```python
from build123d import *

# Parameters (mm, degrees)
SKETCH006_W     = 85.5
SKETCH006_H     = 85.5
SKETCH006_W_2   = 73.5
SKETCH006_H_2   = 73.5
PAD003_DEPTH    = 6
SKETCH007_W     = 85.5
SKETCH007_H     = 85.5
SKETCH007_R     = 25.5
PAD004_DEPTH    = 2
SKETCH008_R     = 1.5
POCKET_DEPTH    = 8.001
SKETCH009_R     = 1.5
POCKET001_DEPTH = 5
FILLET002_R     = 3


with BuildPart() as part:
    # Sketch006 → Pad003 (new body)
    with BuildSketch(Plane.XY):
        Rectangle(SKETCH006_W, SKETCH006_H)
        Rectangle(SKETCH006_W_2, SKETCH006_H_2, mode=Mode.SUBTRACT)
    extrude(amount=PAD003_DEPTH)

    # Sketch007 (on Face10 of Pad003) → Pad004 (join)
    with BuildSketch(Plane.XY.offset(6)):
        Rectangle(SKETCH007_W, SKETCH007_H)
        Circle(SKETCH007_R, mode=Mode.SUBTRACT)
    extrude(amount=PAD004_DEPTH)

    # Sketch008 (on Face4 of Pad004) → Pocket (cut, through all)
    with BuildSketch(Plane(origin=(0, 0, 0), x_dir=(1, 0, 0), z_dir=(0, 0, -1))):
        with Locations((-39.235281, 39.235281)):
            Circle(SKETCH008_R)
        with Locations((39.235281, 39.235281)):
            Circle(SKETCH008_R)
        with Locations((39.235281, -39.235281)):
            Circle(SKETCH008_R)
        with Locations((-39.235281, -39.235281)):
            Circle(SKETCH008_R)
    extrude(amount=-POCKET_DEPTH, mode=Mode.SUBTRACT)

    # Sketch009 (on Face17 of Pocket) → Pocket001 (cut)
    with BuildSketch(Plane.XY.offset(8)):
        with Locations((-30, 30)):
            Circle(SKETCH009_R)
        with Locations((30, 30)):
            Circle(SKETCH009_R)
        with Locations((30, -30)):
            Circle(SKETCH009_R)
        with Locations((-30, -30)):
            Circle(SKETCH009_R)
    extrude(amount=-POCKET001_DEPTH, mode=Mode.SUBTRACT)

    # Fillet002
    fillet002_edges = [part.edges().sort_by_distance(p)[0] for p in [
        (42.75, 42.75, 3),
        (-42.75, 42.75, 3),
        (-42.75, -42.75, 3),
        (42.75, -42.75, 3),
    ]]
    fillet(fillet002_edges, radius=FILLET002_R)


solid = part.part
```
Input: part model. Units: mm. Frame: model coordinates. A direction names the side the tool comes from. Give positions to 0.01 mm unless a question says otherwise; leave off trailing zeros. Write each loop counter-clockwise with the first axis right and the second up, starting at its lowest first coordinate (ties: lowest second). Pieces come first, ordered by that corner, then holes. Notation, with made-up numbers: (-15, -1) - (6, -1) arc R25 ccw to (6, 34) - close; hole circle Ø10 at (-24.5, -10). An arc over 180 degrees is marked (long way). Write item = value, one per line. Start each with the question number.
1. Mould query, pull axis X, two halves, no side actions, for faces 3 (the cylindrical face through (41.85, 41.89, 3.94)), 4 (the flat face through (-1, -42.75, 4)), 5 (the cylindrical face through (-5.5, -24.9, 7)), 6 (the cylindrical face through (-38.43, -40.5, 3.94)). Classes: released by +X, released by -X, zero draft, split by the parting line, or undercut.
2. Section query C-C, the plane x = -30. Output: boundary loops of the cut face in (y, z), then the cut area to 3 significant figures.
3. Section query A-A, the plane x = 0. Output: boundary loops of the cut face in (y, z), then the cut area to 3 significant figures.
4. First-contact query: pin 1 Ø22 at (x, y) = (-0.5, -5.5) entering from -Z; pin 2 Ø3.5 at (x, y) = (-30, -30) entering from -Z. Flat tips, straight axial feed; report the tip coordinate or a pass-through.
5. Ray query, L1, parallel to Y at x = 10.5, z = 3; L2, parallel to Y at x = 30, z = 7. Return the intervals inside material, ascending.
6. Access query for faces 1 (the cylindrical face through (-31.5, 30.07, 7.01)), 2 (the flat face through (36.75, -1, 3)). Directions: +Z, -Z, +X, -X, +Y, -Y. A direction counts if a zero-diameter tool reaches every point of the face in a straight line with its end or side. Return the directions, or none.
Check sheet entries:
q1.face_3 = released by +X
q1.face_4 = zero draft
q1.face_5 = undercut
q1.face_6 = undercut
q2.outline = (-42.75, 0) - (-36.75, 0) - (-36.75, 6) - (-31.5, 6) - (-31.5, 8) - (-42.75, 8) - close; (-28.5, 6) - (28.5, 6) - (28.5, 8) - (-28.5, 8) - close; (31.5, 6) - (36.75, 6) - (36.75, 0) - (42.75, 0) - (42.75, 8) - (31.5, 8) - close
q2.area = 231 mm2
q3.outline = (-42.75, 0) - (-36.75, 0) - (-36.75, 6) - (-25.5, 6) - (-25.5, 8) - (-42.75, 8) - close; (25.5, 6) - (36.75, 6) - (36.75, 0) - (42.75, 0) - (42.75, 8) - (25.5, 8) - close
q3.area = 141 mm2
q4.pin_1 = through
q4.pin_2 = 6
q5.L1 = -42.75 to -36.75, 36.75 to 42.75
q5.L2 = -42.75 to -31.5, -28.5 to 28.5, 31.5 to 42.75
q6.face_1 = +Z, -Z
q6.face_2 = -Z
